Design review of the part built by this model. Coordinates are the model's own, in mm. A direction names the side the tool comes from. Round coordinates to 2 decimals unless told otherwise and drop trailing zeros. Order: outer loops, then holes, each group sorted by start corner. A loop starts at its lowest first (then second) coordinate and runs counter-clockwise, first axis right, second up. Notation, with made-up numbers: (61, 41.5) - (112, 41.5) arc R25 cw to (112, 75.5) - close; hole circle Ø5 at (-30, -31.5). An arc over 180 degrees is marked (long way). Write item = value, one per line.
from build123d import *

# Parameters (mm, degrees)
CROQUIS1_R              = 6.5
SALIENTE_EXTRUIR1_DEPTH = 5
CROQUIS2_W              = 150
CROQUIS2_H              = 76.2
SALIENTE_EXTRUIR2_DEPTH = 5
CROQUIS3_R              = 6.5
CROQUIS3_R_2            = 10
SALIENTE_EXTRUIR3_DEPTH = 5


with BuildPart() as part:
    # Croquis1 → Saliente-Extruir1 (new body)
    with BuildSketch(Plane.XY):
        with BuildLine():
            Line((75, 0), (-75, 0))
            Line((-75, 0), (-21.213203436, 53.786796564))
            ThreePointArc((-21.213203436, 53.786796564), (0, 62.573593129), (21.213203436, 53.786796564))
            Line((21.213203436, 53.786796564), (75, 0))
        make_face()
        with Locations((0, 41.325890401)):
            Circle(CROQUIS1_R, mode=Mode.SUBTRACT)
    extrude(amount=SALIENTE_EXTRUIR1_DEPTH)

    # Croquis2 → Saliente-Extruir2 (add)
    with BuildSketch(Plane.XZ):
        with Locations((0, -33.1)):
            Rectangle(CROQUIS2_W, CROQUIS2_H)
        with BuildLine():
            Line((-38.481595315, -28.1), (-38.481595315, -38.1))
            ThreePointArc((-38.481595315, -38.1), (-45, -44.618404685), (-51.518404685, -38.1))
            Line((-51.518404685, -38.1), (-51.518404685, -28.1))
            ThreePointArc((-51.518404685, -28.1), (-45, -21.581595315), (-38.481595315, -28.1))
        make_face(mode=Mode.SUBTRACT)
        with BuildLine():
            Line((51.37253144, -28.1), (51.37253144, -38.1))
            ThreePointArc((51.37253144, -38.1), (45, -44.47253144), (38.62746856, -38.1))
            Line((38.62746856, -38.1), (38.62746856, -28.1))
            ThreePointArc((38.62746856, -28.1), (45, -21.72746856), (51.37253144, -28.1))
        make_face(mode=Mode.SUBTRACT)
    extrude(amount=SALIENTE_EXTRUIR2_DEPTH)

    # Croquis3 → Saliente-Extruir3 (add)
    with BuildSketch(Plane(origin=(0, 0, 0), x_dir=(-1, 0, 0), z_dir=(0, 0, -1))):
        with BuildLine():
            Line((75, 0), (-58.786796564, 133.786796564))
            ThreePointArc((-58.786796564, 133.786796564), (-80, 142.573593129), (-101.213203436, 133.786796564))
            Line((-101.213203436, 133.786796564), (-101.263160567, 133.736839433))
            ThreePointArc((-101.263160567, 133.736839433), (-110.049957131, 112.523635998), (-101.263160567, 91.310432562))
            Line((-101.263160567, 91.310432562), (-75, 65.047271996))
            Line((-75, 65.047271996), (-75, 0))
            Line((-75, 0), (75, 0))
        make_face()
        with Locations((-80, 115)):
            Circle(CROQUIS3_R, mode=Mode.SUBTRACT)
        with Locations((0, 41.325890401)):
            Circle(CROQUIS3_R_2, mode=Mode.SUBTRACT)
    extrude(amount=-SALIENTE_EXTRUIR3_DEPTH)


solid = part.part
Item 1: Take a section at D-D, the plane z = -16.5. State the section outline as (x, y) points.
Data:
outline = (-75, -5) - (75, -5) - (75, 0) - (-75, 0) - close
Item 2: Take a section at B-B, the plane y = 115. State the section outline as (x, z) points, and give its area (3 significant figures).
Data:
outline = (40, 0) - (73.5, 0) - (73.5, 5) - (40, 5) - close; (86.5, 0) - (109.95, 0) - (109.95, 5) - (86.5, 5) - close
area = 285 mm2
Item 3: For line 1 along Y through (x, z) = (0, 2.35); line 2 along Z through (x, y) = (-9.5, 14.5); line 3 along Y through (x, z) = (-25.5, -42), list the stretches that pass through material, from the lowest coordinate up. Write a range as [from, to].
Data:
line_1 = [-5, 34.83], [47.83, 75]
line_2 = [0, 5]
line_3 = [-5, 0]
Item 4: Insertion check: P1, Ø8, axis at x = 80, y = 115, coming from the +Z side; P2, Ø4, axis at y = -2, z = -34, coming from the +X side; P3, Ø3, axis at x = -39.5, z = -41, coming from the +Y side; P4, Ø6, axis at x = 35, y = 93, coming from the -Z side. Each pin has a flat end and moves straight along its axis. Give the tip position at first contact, or say it passes through.
Data:
P1 = through
P2 = 75
P3 = 0
P4 = 0
Item 5: For faces 4 (the face through (75, -1, -16)), 5 (the face through (-1, 0, -35)), 6 (the face through (-44.857, -2.465, -44.617)), list the 3-axis set-ups (+Z, -Z, +X, -X, +Y, -Y) from which the entire face can be reached by the end or side of a thin tool; tool diameter is ignored.
Data:
face_4 = +Z, -Z, +X, -Y
face_5 = -Z, +X, -X, +Y
face_6 = +Y, -Y
Item 6: Take a section at C-C, the plane x = -45. State the section outline as (y, z) points, and give its area (3 significant figures).
Data:
outline = (-5, -71.2) - (0, -71.2) - (0, -44.62) - (-5, -44.62) - close; (-5, -21.58) - (0, -21.58) - (0, 0) - (30, 0) - (30, 5) - (-5, 5) - close
area = 416 mm2
Item 7: Take a section at A-A, the plane x = 0. State the section outline as (y, z) points, and give its area (3 significant figures).
Data:
outline = (-5, -71.2) - (0, -71.2) - (0, 0) - (34.83, 0) - (34.83, 5) - (-5, 5) - close; (47.83, 0) - (75, 0) - (75, 5) - (47.83, 5) - close
area = 691 mm2
Item 8: The part is to be moulded in two halves that separate along Y. For faces 1 (the face through (51.373, -2, -33)), 2 (the face through (88.315, 78.363, 2.465)), 3 (the face through (3, 35.56, 2.46)), say which applies: +Y half, -Y half, draft (parallel to the pull), parting line (faces both ways), or undercut.
Data:
face_1 = draft
face_2 = -Y half
face_3 = undercut
